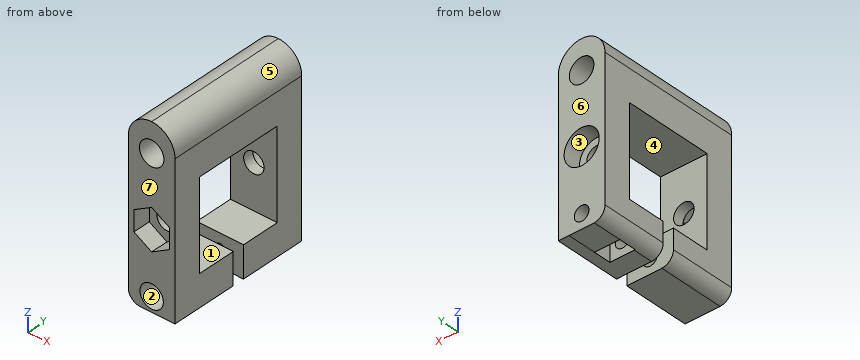
Autodesk Inventor part; units mm, degrees
ref_plane "YZ Plane" through (0, 0, 0) normal (1, 0, 0) x (0, 1, 0)
ref_plane "XZ Plane" through (0, 0, 0) normal (0, 1, 0) x (-1, 0, 0)
ref_plane "XY Plane" through (0, 0, 0) normal (0, 0, 1) x (1, 0, 0)
sketch "Sketch1" plane through (0, 0, 0) normal (1, 0, 0) x (0, 1, 0)
  line L0 (-12.4, 15) -> (12.4, 15)
  line L1 (12.4, 15) -> (12.4, -15)
  line L2 (12.4, -15) -> (-12.4, -15)
  line L3 (-12.4, -15) -> (-12.4, 15)
  line L4 (-12.4, 15) -> (12.4, -15) construction
  line L5 (12.4, 15) -> (-12.4, -15) construction
  line L6 (0, -15) -> (0, -1.5)
  circle A0 centre (0, -1.5) radius 8
  point P0 (0, 0)
  dimension "d0" = 24.8
  dimension "d1" = 30
  dimension "d2" = 13.5
  dimension "d3" = 16
extrude "Extrusion1" add sketch "Sketch1" along normal blind 8
sketch "Sketch3" plane through (0, 12.4, 15) normal (0, 1, 0) x (1, 0, 0)
  line L0 (0, 0) -> (8, 0)
  line L1 (4, 0) -> (4, 5)
  circle A0 centre (4, 5) radius 2.1
  point P0 (0, 15)
  dimension "d9" = 5
  dimension "d10" = 4.2
extrude "Extrusion3" cut sketch "Sketch3" against normal up to next
sketch "Sketch4" plane through (0, 12.4, 15) normal (0, 1, 0) x (1, 0, 0)
  line L0 (0, 30) -> (8, 30)
  line L1 (4, 30) -> (4, 27.5)
  circle A0 centre (4, 27.5) radius 1.25
  point P0 (0, 15)
  dimension "d13" = 2.5
  dimension "d14" = 2.5
extrude "Extrusion4" cut sketch "Sketch4" against normal through all
fillet "Fillet1" radius 4 2 edges at (0, 0, 15) (8, 0, 15)
fillet "Fillet2" radius 2 1 edges at (0, 0, -15)
sketch "Sketch5" plane through (8, 0, 0) normal (1, 0, 0) x (0, 0, -1)
  arc A0 (1.5, 8) -> (1.5, 8) centre (1.5, 0) ccw
  circle A1 centre (1.5, 0) radius 8
  point P0 (0, 0)
extrude "Extrusion5" add sketch "Sketch5" against normal blind 8
sketch "Sketch6" plane through (8, 0, 0) normal (1, 0, 0) x (0, 0, -1)
  line L0 (-5.6, -7.6) -> (9.6, -7.6)
  line L1 (9.6, -7.6) -> (9.6, 7.6)
  line L2 (9.6, 7.6) -> (-5.6, 7.6)
  line L3 (-5.6, 7.6) -> (-5.6, -7.6)
  line L4 (-5.6, -7.6) -> (9.6, 7.6) construction
  line L5 (9.6, -7.6) -> (-5.6, 7.6) construction
  point P0 (0, 0)
  point P1 (2, 0)
  dimension "d22" = 15.2
  dimension "d23" = 15.2
  dimension "d24" = 2
extrude "Extrusion6" cut sketch "Sketch6" against normal up to next
sketch "Sketch7" plane through (8, 0, 0) normal (1, 0, 0) x (0, 0, -1)
  line L0 (8.4724, -1) -> (16.4136, -1)
  line L1 (16.4136, -1) -> (16.4136, 1)
  line L2 (16.4136, 1) -> (8.4724, 1)
  line L3 (8.4724, 1) -> (8.4724, -1)
  line L4 (8.4724, -1) -> (16.4136, 1) construction
  line L5 (16.4136, -1) -> (8.4724, 1) construction
  point P0 (0, 0)
  point P1 (12.443, 0)
  dimension "d27" = 2
extrude "Extrusion7" cut sketch "Sketch7" against normal through all
sketch "Sketch8" plane through (4, 12.4, 11) normal (0, 1, 0) x (1, 0, 0)
  circle A0 centre (0, 23.5) radius 1.25
  line L0 (0, 26) -> (2.1651, 24.75)
  line L1 (2.1651, 24.75) -> (2.1651, 22.25)
  line L2 (2.1651, 22.25) -> (0, 21)
  line L3 (0, 21) -> (-2.1651, 22.25)
  line L4 (-2.1651, 22.25) -> (-2.1651, 24.75)
  line L5 (-2.1651, 24.75) -> (0, 26)
  point P0 (-4, 11)
  dimension "d30" = 2.5
extrude "Extrusion8" cut sketch "Sketch8" against normal blind 8
sketch "Sketch9" plane through (4, 4.4, -10) normal (0.5, 0, -0.8660254) x (-0.8660254, 0, -0.5)
  point P0 (-1.5359, -4.4)
sketch "Sketch10" plane through (4, 12.4, 11) normal (0, 1, 0) x (1, 0, 0)
  line L0 (-2.1651, 24.75) -> (0, 26)
  line L1 (2.1651, 27.25) -> (-2.1651, 27.25)
  line L2 (-2.1651, 27.25) -> (-2.1651, 24.75)
  line L3 (-2.1651, 24.75) -> (2.1651, 24.75)
  line L4 (2.1651, 24.75) -> (2.1651, 27.25)
  line L5 (0, 26) -> (2.1651, 24.75)
  line L6 (2.1651, 27.25) -> (-2.1651, 24.75) construction
  line L7 (-2.1651, 27.25) -> (2.1651, 24.75) construction
  point P0 (-4, 11)
extrude "Extrusion9" cut sketch "Sketch10" against normal blind 8
sketch "Sketch11" plane through (4, 12.4, 11) normal (0, 1, 0) x (1, 0, 0)
  line L0 (2.1651, 22.25) -> (0, 21)
  line L1 (0, 21) -> (-2.1651, 22.25)
  arc A0 (-2.1651, 25.9932) -> (-4, 24) centre (-2, 24) ccw
  line L2 (-4, 24) -> (-2.1651, 22.25)
  arc A1 (-2.1651, 25.9932) -> (-4, 24) centre (-2, 24) ccw
  line L3 (-2.1651, 25.9932) -> (2.1651, 26)
  line L4 (2.1651, 22.25) -> (0, 21)
  line L5 (2.1651, 26) -> (2.1651, 22.25)
  line L6 (2.1651, 22.25) -> (0, 21)
  circle A2 centre (0, 23.5) radius 1.25
  circle A3 centre (0, 23.5) radius 1.25
  point P0 (-4, 11)
extrude "Extrusion10" add sketch "Sketch11" against normal blind 5
sketch "Sketch12" plane through (4, -12.4, 11) normal (0, -1, 0) x (1, 0, 0)
  circle A0 centre (0, -23.5) radius 1.25
  circle A1 centre (0, -23.5) radius 2
  point P0 (-4, -11)
  dimension "d37" = 4
extrude "Extrusion11" cut sketch "Sketch12" against normal blind 4
sketch "Sketch13" plane through (4, 12.4, 11) normal (0, 1, 0) x (1, 0, 0)
  line L0 (-2, 26) -> (4, 26)
  line L1 (4, 26) -> (0, 26)
  line L2 (0, 26) -> (0, 13)
  line L3 (0, 13) -> (4, 13)
  line L4 (4, 13) -> (4, 26)
  circle A0 centre (0, 13) radius 1.75
  point P0 (-4, 11)
  dimension "d40" = 4
  dimension "d41" = 13
  dimension "d42" = 3.5
extrude "Extrusion12" cut sketch "Sketch13" against normal through all contours A0 L3 L2 | L2 L3 A0
sketch "Sketch14" plane through (4, -12.4, 11) normal (0, -1, 0) x (1, 0, 0)
  circle A0 centre (0, -13) radius 1.75
  line L0 (0, -16.5) -> (-3.0311, -14.75)
  line L1 (-3.0311, -14.75) -> (-3.0311, -11.25)
  line L2 (-3.0311, -11.25) -> (0, -9.5)
  line L3 (0, -9.5) -> (3.0311, -11.25)
  line L4 (3.0311, -11.25) -> (3.0311, -14.75)
  line L5 (3.0311, -14.75) -> (0, -16.5)
  point P0 (-4, -11)
  dimension "d45" = 3.5
extrude "Extrusion13" cut sketch "Sketch14" against normal blind 3
sketch "Sketch15" plane through (4, 12.4, 11) normal (0, 1, 0) x (1, 0, 0)
  circle A0 centre (0, 13) radius 1.75
  circle A1 centre (0, 13) radius 3
  point P0 (-4, 11)
  dimension "d48" = 6
extrude "Extrusion14" cut sketch "Sketch15" against normal blind 3
properties part number "arm_grip" material "Nylon 6/6"
The listing builds one solid part. Answer for the finished solid, in the listing's coordinates (mm). Face numbers are marked on the shaded views. A direction names the side the tool comes from. Coordinates: 2 decimals unless noted, no trailing zeros. Write each loop counter-clockwise with the first axis right and the second up, starting at its lowest first coordinate (ties: lowest second). Pieces come first, ordered by that corner, then holes. Notation, with made-up numbers: (-3.5, 87) -> (6.5, 87) arc R19 ccw to (6.5, 100) -> close; hole circle Ø2 at (38, 45). An arc over 180 degrees is marked (long way). Write each question's results on one line, items separated by ' | '. Start each with the question number.
1) A cutting plane is placed at C-C (z = -2). Determine the outline of the cut face in (x, y), then the cut area to 3 significant figures.
2) A tool of negligible diameter and unlimited length cuts with its end or side. For the marked faces 1, 2 and 3, from which of +Z, -Z, +X, -X, +Y, -Y can it reach the whole face along a straight path? Write none if from no direction.
3) A cutting plane is placed at D-D (z = 10). Determine the outline of the cut face in (x, y), then the cut area to 3 significant figures.
4) Flat-ended cylindrical pins translate along their axes: pin 1 Ø4 at (x, z) = (4, 10) entering from -Y; pin 2 Ø2.5 at (x, z) = (5.5, -2.5) entering from +Y; pin 3 Ø1.6 at (x, z) = (3.5, -13.5) entering from -Y. Find the tip coordinate at first contact, or state that the pin passes through.
5) For a pull along Y with two mould halves and no side action, classify the marked faces 4, 5, 6 and 7 as +Y half, -Y half, draft (parallel to the pull), parting line (faces both ways), or undercut.
6) A cutting plane is placed at B-B (z = -9). Determine the outline of the cut face in (x, y).
7) Straight lines are drawn through the part: probe 1 along Z at (x, y) = (4, -8); probe 2 along Z at (x, y) = (4, 11.2); probe 3 along Y at (x, z) = (7.5, -6). For each, find the intervals that lie inside material, in ascending order.
8) A cutting plane is placed at A-A (y = 3.5). Count the separate pieces of the cut face and the enclosed holes in it, then the cut area to 3 significant figures.
Values follow:
1) outline: (0, -12.4) -> (0.97, -12.4) -> (0.97, -9.4) -> (2.25, -9.4) -> (2.25, -7.6) -> (0, -7.6) -> close; (0, 7.6) -> (2.25, 7.6) -> (2.25, 9.4) -> (1, 9.4) -> (1, 12.4) -> (0, 12.4) -> close; (5.75, -9.4) -> (7.03, -9.4) -> (7.03, -12.4) -> (8, -12.4) -> (8, -7.6) -> (5.75, -7.6) -> close; (5.75, 7.6) -> (8, 7.6) -> (8, 12.4) -> (7, 12.4) -> (7, 9.4) -> (5.75, 9.4) -> close | area: 28.0 mm²
2) face 1: +X, -X | face 2: -Y | face 3: +Y
3) outline: (0, -12.4) -> (1.9, -12.4) -> (1.9, 12.4) -> (0, 12.4) -> close; (6.1, -12.4) -> (8, -12.4) -> (8, 12.4) -> (6.1, 12.4) -> close | area: 94.2 mm²
4) pin 1: through | pin 2: y = 9.4 | pin 3: y = -8.4
5) face 4: undercut | face 5: draft | face 6: +Y half | face 7: -Y half
6) outline: (0, -12.4) -> (8, -12.4) -> (8, -7.6) -> (0, -7.6) -> close; (0, 7.6) -> (8, 7.6) -> (8, 12.4) -> (0, 12.4) -> close
7) probe 1: -15 to -13.75, -11.25 to -3.75, -0.25 to 7.9, 12.1 to 15 | probe 2: -15 to -13.75, -11.25 to -5, 1 to 7.9, 12.1 to 15 | probe 3: -12.4 to -7.6, 7.6 to 12.4
8) separate pieces: 2 | enclosed holes: 2 | area: 91.9 mm²
